The listing builds one solid part. Answer for the finished solid, in the listing's coordinates (mm). Face numbers are marked on the shaded views. Round coordinates to 2 decimals unless told otherwise and drop trailing zeros. Write each loop counter-clockwise with the first axis right and the second up, starting at its lowest first coordinate (ties: lowest second). Pieces come first, ordered by that corner, then holes. Notation, with made-up numbers: (-29.75, 80) - (25.25, 80) arc R21 ccw to (25.25, 108) - close; hole circle Ø10 at (61, 84.5). An arc over 180 degrees is marked (long way). Use a Markdown table: item, result. Add a question column.
1) A cutting plane is placed at D-D (z = 17.68). Give the vertices of the cut face in (x, y) (3 decimals), then the cut area to 3 significant figures.
2) A cutting plane is placed at A-A (y = 3). State how many separate pieces and enclosed holes the cut face has, then the cut area to 3 significant figures.
3) Find the intervals of material crossed by probe 1 along X at (y, z) = (4, -17.68) (3 decimals); probe 2 along Z at (x, y) = (15, 6.5); probe 3 along Z at (x, y) = (29, 7), in increasing order. Write a range as from..to.
4) Each of these flat-tipped pins is pushed along its axis until it touches: P1, Ø4, axis at x = 17.8, z = 7.6, coming from the -Y side; P2, Ø1.5, axis at y = -2, z = -31.5, coming from the +X side; P3, Ø4, axis at y = -3.5, z = -31.5, coming from the -X side. Where does it stop, or does it pass through?
5) Determine the mould class of the marked faces 1, 2, 3 and 4 for opening direction Z: +Z half, -Z half, draft (parallel to the pull), parting line (faces both ways), or undercut.
6) A cutting plane is placed at B-B (z = -7.6). Give the vertices of the cut face in (x, y) (3 decimals), then the cut area to 3 significant figures.
```python
from build123d import *

# Parameters (mm, degrees)
BOSS_EXTRUDE1_DEPTH = 8
SKETCH2_W           = 7
SKETCH2_H           = 12
SKETCH2_R           = 1.775
SKETCH2_W_2         = 12
SKETCH2_H_2         = 7
BOSS_EXTRUDE2_DEPTH = 13
SKETCH7_R           = 1.775
CUT_EXTRUDE1_DEPTH  = 55.603113464
FILLET1_R           = 1
SKETCH9_R           = 1.525
CUT_EXTRUDE3_DEPTH  = 55.603113464
CUT_EXTRUDE4_DEPTH  = 3.6
SKETCH12_R          = 5.525
CUT_EXTRUDE5_DEPTH  = 55.603113464
BOSS_EXTRUDE3_DEPTH = 12
FILLET2_R           = 2


with BuildPart() as part:
    # Sketch1 → Boss-Extrude1 (new body)
    with BuildSketch(Plane(origin=(0, 0, 0), x_dir=(1, 0, 0), z_dir=(0, 1, 0))):
        with BuildLine():
            Line((35.5, -37.5), (-35.5, -37.5))
            ThreePointArc((-35.5, -37.5), (-36.914213562, -36.914213562), (-37.5, -35.5))
            Line((-37.5, -35.5), (-37.5, 35.5))
            ThreePointArc((-37.5, 35.5), (-36.914213562, 36.914213562), (-35.5, 37.5))
            Line((-35.5, 37.5), (35.5, 37.5))
            ThreePointArc((35.5, 37.5), (36.914213562, 36.914213562), (37.5, 35.5))
            Line((37.5, 35.5), (37.5, -35.5))
            ThreePointArc((37.5, -35.5), (36.914213562, -36.914213562), (35.5, -37.5))
        make_face()
    extrude(amount=BOSS_EXTRUDE1_DEPTH)

    # Sketch2 → Boss-Extrude2 (add)
    # profile 1 of 4: a face of its own
    with BuildSketch(Plane(origin=(0, 8, 0), x_dir=(1, 0, 0), z_dir=(0, 1, 0))):
        with Locations((-31.5, -29)):
            Rectangle(SKETCH2_W, SKETCH2_H)
        with Locations(Location((-31.5, -26, 0), (0, 0, 270))):
            Circle(SKETCH2_R, mode=Mode.SUBTRACT)
        with Locations(Location((-31.5, -32, 0), (0, 0, 270))):
            Circle(SKETCH2_R, mode=Mode.SUBTRACT)
    # profile 2 of 4: a face of its own
    with BuildSketch(Plane(origin=(0, 8, 0), x_dir=(1, 0, 0), z_dir=(0, 1, 0))):
        with Locations((29, -31.5)):
            Rectangle(SKETCH2_W_2, SKETCH2_H_2)
        with Locations(Location((26, -31.5, 0), (0, 0, 270))):
            Circle(SKETCH2_R, mode=Mode.SUBTRACT)
        with Locations(Location((32, -31.5, 0), (0, 0, 270))):
            Circle(SKETCH2_R, mode=Mode.SUBTRACT)
    # profile 3 of 4: a face of its own
    with BuildSketch(Plane(origin=(0, 8, 0), x_dir=(1, 0, 0), z_dir=(0, 1, 0))):
        with Locations((31.5, 29)):
            Rectangle(SKETCH2_W, SKETCH2_H)
        with Locations(Location((31.5, 26, 0), (0, 0, 270))):
            Circle(SKETCH2_R, mode=Mode.SUBTRACT)
        with Locations(Location((31.5, 32, 0), (0, 0, 270))):
            Circle(SKETCH2_R, mode=Mode.SUBTRACT)
    # profile 4 of 4: a face of its own
    with BuildSketch(Plane(origin=(0, 8, 0), x_dir=(1, 0, 0), z_dir=(0, 1, 0))):
        with Locations((-29, 31.5)):
            Rectangle(SKETCH2_W_2, SKETCH2_H_2)
        with Locations(Location((-26, 31.5, 0), (0, 0, 270))):
            Circle(SKETCH2_R, mode=Mode.SUBTRACT)
        with Locations(Location((-32, 31.5, 0), (0, 0, 270))):
            Circle(SKETCH2_R, mode=Mode.SUBTRACT)
    extrude(amount=-BOSS_EXTRUDE2_DEPTH)

    # Sketch7 → Cut-Extrude1 (cut, through all)
    with BuildSketch(Plane(origin=(0, 8, 0), x_dir=(1, 0, 0), z_dir=(0, 1, 0))):
        with Locations(Location((32, -31.5, 0), (0, 0, 270))):
            Circle(SKETCH7_R)
        with Locations(Location((26, -31.5, 0), (0, 0, 270))):
            Circle(SKETCH7_R)
        with Locations(Location((-31.5, -32, 0), (0, 0, 270))):
            Circle(SKETCH7_R)
        with Locations(Location((-31.5, -26, 0), (0, 0, 270))):
            Circle(SKETCH7_R)
        with Locations(Location((31.5, 26, 0), (0, 0, 270))):
            Circle(SKETCH7_R)
        with Locations(Location((31.5, 32, 0), (0, 0, 270))):
            Circle(SKETCH7_R)
        with Locations(Location((-26, 31.5, 0), (0, 0, 270))):
            Circle(SKETCH7_R)
        with Locations(Location((-32, 31.5, 0), (0, 0, 270))):
            Circle(SKETCH7_R)
    extrude(amount=-CUT_EXTRUDE1_DEPTH, mode=Mode.SUBTRACT)

    # Fillet1
    fillet1_edges = [part.edges().sort_by_distance(p)[0] for p in [
        (35, -2.5, -35),
        (35, -2.5, -23),
        (28, -2.5, -23),
        (28, -2.5, -35),
        (35, -2.5, 28),
        (35, -2.5, 35),
        (23, -2.5, 35),
        (23, -2.5, 28),
        (-35, -2.5, 35),
        (-35, -2.5, 23),
        (-28, -2.5, 23),
        (-28, -2.5, 35),
        (-35, -2.5, -28),
        (-35, -2.5, -35),
        (-23, -2.5, -35),
        (-23, -2.5, -28),
    ]]
    fillet(fillet1_edges, radius=FILLET1_R)

    # Sketch9 → Cut-Extrude3 (cut, through all)
    with BuildSketch(Plane(origin=(0, 8, 0), x_dir=(1, 0, 0), z_dir=(0, 1, 0))):
        with Locations(Location((-17.8, 7.6, 0), (0, 0, 270))):
            Circle(SKETCH9_R)
        with Locations(Location((17.8, 7.6, 0), (0, 0, 270))):
            Circle(SKETCH9_R)
        with Locations(Location((-17.8, -7.6, 0), (0, 0, 270))):
            Circle(SKETCH9_R)
        with Locations(Location((17.8, -7.6, 0), (0, 0, 270))):
            Circle(SKETCH9_R)
    extrude(amount=-CUT_EXTRUDE3_DEPTH, mode=Mode.SUBTRACT)

    # Sketch11 → Cut-Extrude4 (cut)
    with BuildSketch(Plane(origin=(0, 8, 0), x_dir=(1, 0, 0), z_dir=(0, 1, 0))):
        with BuildLine():
            Line((-32, 34.9), (-26, 34.9))
            ThreePointArc((-26, 34.9), (-22.6, 31.5), (-26, 28.1))
            Line((-26, 28.1), (-32, 28.1))
            ThreePointArc((-32, 28.1), (-35.4, 31.5), (-32, 34.9))
        make_face()
        with BuildLine():
            Line((-28.1, -26), (-28.1, -32))
            ThreePointArc((-28.1, -32), (-31.5, -35.4), (-34.9, -32))
            Line((-34.9, -32), (-34.9, -26))
            ThreePointArc((-34.9, -26), (-31.5, -22.6), (-28.1, -26))
        make_face()
        with BuildLine():
            Line((26, -28.1), (32, -28.1))
            ThreePointArc((32, -28.1), (35.4, -31.5), (32, -34.9))
            Line((32, -34.9), (26, -34.9))
            ThreePointArc((26, -34.9), (22.6, -31.5), (26, -28.1))
        make_face()
        with BuildLine():
            Line((34.9, 32), (34.9, 26))
            ThreePointArc((34.9, 26), (31.5, 22.6), (28.1, 26))
            Line((28.1, 26), (28.1, 32))
            ThreePointArc((28.1, 32), (31.5, 35.4), (34.9, 32))
        make_face()
    extrude(amount=-CUT_EXTRUDE4_DEPTH, mode=Mode.SUBTRACT)

    # Sketch12 → Cut-Extrude5 (cut, through all)
    with BuildSketch(Plane(origin=(0, 8, 0), x_dir=(1, 0, 0), z_dir=(0, 1, 0))):
        with Locations(Location((-17.68, 17.68, 0), (0, 0, 270))):
            Circle(SKETCH12_R)
        with Locations(Location((-17.68, -17.68, 0), (0, 0, 270))):
            Circle(SKETCH12_R)
        with Locations(Location((17.68, -17.68, 0), (0, 0, 270))):
            Circle(SKETCH12_R)
        with Locations(Location((17.68, 17.68, 0), (0, 0, 270))):
            Circle(SKETCH12_R)
    extrude(amount=-CUT_EXTRUDE5_DEPTH, mode=Mode.SUBTRACT)

    # Sketch13 → Boss-Extrude3 (add)
    with BuildSketch(Plane(origin=(0, 8, 0), x_dir=(1, 0, 0), z_dir=(0, 1, 0))):
        with BuildLine():
            Line((1, -2), (-1, -2))
            ThreePointArc((-1, -2), (-1.707106781, -1.707106781), (-2, -1))
            Line((-2, -1), (-2, 1))
            ThreePointArc((-2, 1), (-1.707106781, 1.707106781), (-1, 2))
            Line((-1, 2), (1, 2))
            ThreePointArc((1, 2), (1.707106781, 1.707106781), (2, 1))
            Line((2, 1), (2, -1))
            ThreePointArc((2, -1), (1.707106781, -1.707106781), (1, -2))
        make_face()
    extrude(amount=BOSS_EXTRUDE3_DEPTH)

    # Fillet2
    fillet2_edges = [part.edges().sort_by_distance(p)[0] for p in [
        (-1.707106781, 8, 1.707106781),
        (0, 8, 2),
        (1.707106781, 8, 1.707106781),
        (2, 8, 0),
        (1.707106781, 8, -1.707106781),
        (0, 8, -2),
        (-1.707106781, 8, -1.707106781),
        (-2, 8, 0),
    ]]
    fillet(fillet2_edges, radius=FILLET2_R)


solid = part.part
```
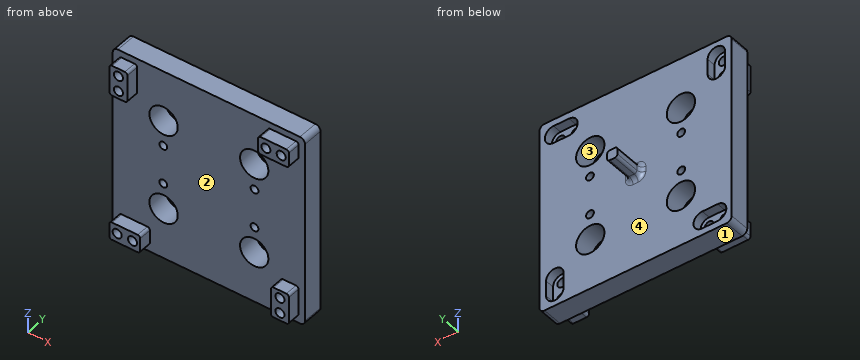
Entries:
| question | item | result |
|---|---|---|
| 1 | outline | (-37.5, 0) - (-23.205, 0) - (-23.205, 8) - (-37.5, 8) - close; (-12.155, 0) - (12.155, 0) - (12.155, 8) - (-12.155, 8) - close; (23.205, 0) - (37.5, 0) - (37.5, 8) - (23.205, 8) - close |
| 1 | area | 423 mm² |
| 2 | separate pieces | 1 |
| 2 | enclosed holes | 16 |
| 2 | area | 5,130 mm² |
| 3 | probe 1 | x = -37.5..-23.205, -12.155..12.155, 23.205..37.5 |
| 3 | probe 2 | z = -37.5..-22.51, -12.85..12.85, 22.51..37.5 |
| 3 | probe 3 | z = -37.5..-34.3, -23.7..28.1, 34.9..37.5 |
| 4 | P1 | stops at y = 0 |
| 4 | P2 | stops at x = 35 |
| 4 | P3 | stops at x = -35 |
| 5 | face 1 | -Z half |
| 5 | face 2 | undercut |
| 5 | face 3 | undercut |
| 5 | face 4 | draft |
| 6 | outline | (-37.5, 0) - (-19.325, 0) - (-19.325, 8) - (-37.5, 8) - close; (-16.275, 0) - (16.275, 0) - (16.275, 8) - (-16.275, 8) - close; (19.325, 0) - (37.5, 0) - (37.5, 8) - (19.325, 8) - close |
| 6 | area | 551 mm² |
